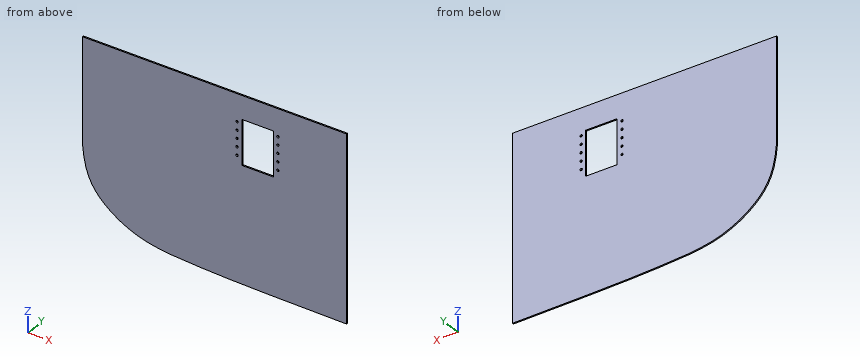
```python
from build123d import *

# Parameters (mm, degrees)
CROQUIS1_R              = 2
CROQUIS1_W              = 54.1
CROQUIS1_H              = 76.7
SALIENTE_EXTRUIR1_DEPTH = 2.4


with BuildPart() as part:
    # Croquis1 → Saliente-Extruir1 (new body)
    with BuildSketch(Plane(origin=(0, 0, 0), x_dir=(1, 0, 0), z_dir=(0, 1, 0))):
        with BuildLine():
            Line((-226.279027723, 0), (226.279027723, 0))
            Line((226.279027723, 0), (226.279027723, 317))
            add(Edge.make_bspline(
                [(226.279027723, 317), (126.058596011, 315.530489859), (25.957083457, 316.912644391), (-74, 309.175657787)],
                knots=[0, 0, 0, 0, 1, 1, 1, 1], degree=3))
            add(Edge.make_bspline(
                [(-226.279027723, 180), (-223.667205932, 215.476583649), (-213.411911356, 241.728935898), (-180.591001989, 273.897889753), (-156.350341436, 289.269961958), (-113.067752708, 305.04715057), (-89.421541744, 307.637409523), (-74, 309.175657787)],
                knots=[0, 0, 0, 0, 0.358064893, 0.430060637, 0.687746689, 0.747961701, 1, 1, 1, 1], degree=3))
            Line((-226.279027723, 180), (-226.279027723, 0))
        make_face()
        with Locations(Location((38.679027723, 102.7, 0), (0, 0, 270))):
            Circle(CROQUIS1_R, mode=Mode.SUBTRACT)
        with Locations(Location((108.679027723, 102.7, 0), (0, 0, 270))):
            Circle(CROQUIS1_R, mode=Mode.SUBTRACT)
        with Locations(Location((108.679027723, 88.7, 0), (0, 0, 270))):
            Circle(CROQUIS1_R, mode=Mode.SUBTRACT)
        with Locations(Location((108.679027723, 74.7, 0), (0, 0, 270))):
            Circle(CROQUIS1_R, mode=Mode.SUBTRACT)
        with Locations(Location((108.679027723, 60.7, 0), (0, 0, 270))):
            Circle(CROQUIS1_R, mode=Mode.SUBTRACT)
        with Locations(Location((108.679027723, 46.7, 0), (0, 0, 270))):
            Circle(CROQUIS1_R, mode=Mode.SUBTRACT)
        with Locations(Location((38.679027723, 88.7, 0), (0, 0, 270))):
            Circle(CROQUIS1_R, mode=Mode.SUBTRACT)
        with Locations(Location((38.679027723, 74.7, 0), (0, 0, 270))):
            Circle(CROQUIS1_R, mode=Mode.SUBTRACT)
        with Locations(Location((38.679027723, 60.7, 0), (0, 0, 270))):
            Circle(CROQUIS1_R, mode=Mode.SUBTRACT)
        with Locations(Location((38.679027723, 46.7, 0), (0, 0, 270))):
            Circle(CROQUIS1_R, mode=Mode.SUBTRACT)
        with Locations((74.229027723, 78.35)):
            Rectangle(CROQUIS1_W, CROQUIS1_H, mode=Mode.SUBTRACT)
    extrude(amount=SALIENTE_EXTRUIR1_DEPTH)


solid = part.part
```
Geometry check sheet. Reference: the model listing, model coordinates, mm. Coordinates: 2 decimals unless noted, no trailing zeros. Use CSV: the item, a comma, the result in double quotes. Start each with the question number.
Item 1: Thickness scan on line 1 (X direction, y = 0.65, z = -74.7); line 2 (X direction, y = 2, z = -73.5); line 3 (X direction, y = 1, z = -49.5). Record the ranges inside material, lowest first.
Item 2: Depth check by flat-ended pin: pin 1 Ø5 at (x, z) = (108.68, -60.7) entering from -Y; pin 2 Ø1 at (x, y) = (-170, 1.5) entering from -Z. Enter the tip coordinate at first touch or a pass-through.
Item 3: Cross-section at A-A, the plane y = 0.8. State how many separate pieces and enclosed holes the cut face has, plus the area to 3 significant figures.
Answers:
1,line 1,"-226.28 to 36.68, 40.68 to 47.18, 101.28 to 106.68, 110.68 to 226.28"
1,line 2,"-226.28 to 37.08, 40.28 to 47.18, 101.28 to 107.08, 110.28 to 226.28"
1,line 3,"-226.28 to 47.18, 101.28 to 226.28"
2,pin 1,"y = 0"
2,pin 2,"z = -279.99"
3,separate pieces,"1"
3,enclosed holes,"11"
3,area,"133,000 mm^2"
